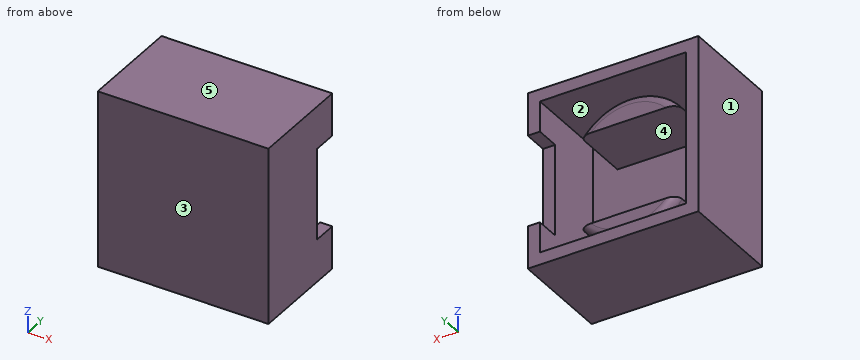
```python
from build123d import *

# Parameters (mm, degrees)
SKETCH1_W            = 30.48
SKETCH1_H            = 31.75
BOSS_EXTRUDE1_DEPTH  = 3.556
BOSS_EXTRUDE2_DEPTH  = 12.7
SKETCH4_W            = 69.596
SKETCH4_H            = 73.406
BOSS_EXTRUDE3_DEPTH  = 3.556
BOSS_EXTRUDE5_DEPTH  = 12.7
MIRROR2_COPY_1_DEPTH = 12.7
MIRROR4_COPY_1_DEPTH = 12.7
FILLET5_R            = 1.778
BOSS_EXTRUDE7_REACH  = 82.336
SKETCH9_W            = 1.524
SKETCH9_H            = 35.306
SKETCH9_H_2          = 2.794
SKETCH9_W_2          = 34.036
CUT_EXTRUDE1_DEPTH   = 81.335506123
SKETCH11_W           = 35.56
SKETCH11_H           = 36.83
SKETCH11_W_2         = 34.036
SKETCH11_H_2         = 35.306
BOSS_EXTRUDE8_DEPTH  = 16.256
BOSS_EXTRUDE9_DEPTH  = 5.08


with BuildPart() as part:
    # Sketch1 → Boss-Extrude1 (new body)
    with BuildSketch(Plane(origin=(0, 0, 0), x_dir=(1, 0, 0), z_dir=(0, 1, 0))):
        with Locations((15.24, 15.875)):
            Rectangle(SKETCH1_W, SKETCH1_H)
    extrude(amount=BOSS_EXTRUDE1_DEPTH)

    # Sketch2 → Boss-Extrude2 (add)
    with BuildSketch(Plane(origin=(0, 3.556, 0), x_dir=(1, 0, 0), z_dir=(0, 1, 0))):
        with BuildLine():
            Line((25.4, 6.35), (5.08, 6.35))
            ThreePointArc((5.08, 6.35), (15.24, 1.27), (25.4, 6.35))
        make_face()
        with BuildLine():
            ThreePointArc((25.4, 25.4), (15.24, 30.48), (5.08, 25.4))
            Line((5.08, 25.4), (25.4, 25.4))
        make_face()
    boss_extrude2 = extrude(amount=BOSS_EXTRUDE2_DEPTH)

    # Sketch4 → Boss-Extrude3 (add)
    with BuildSketch(Plane(origin=(0, 3.556, 0), x_dir=(1, 0, 0), z_dir=(0, 1, 0))):
        with Locations((33.02, -3.175)):
            Rectangle(SKETCH4_W, SKETCH4_H)
    extrude(amount=-BOSS_EXTRUDE3_DEPTH)

    # Sketch8 → Boss-Extrude5 (add)
    with BuildSketch(Plane(origin=(0, 3.556, 0), x_dir=(1, 0, 0), z_dir=(0, 1, 0))):
        Polygon((-1.778, 33.528), (-1.778, 27.178), (-1.778, 4.572), (-1.778, -1.778), (32.258, -1.778), (32.258, 33.528), align=None)
        Polygon((0, 27.178), (0, 31.75), (30.48, 31.75), (30.48, 0), (0, 0), (0, 4.572), align=None, mode=Mode.SUBTRACT)
    boss_extrude5 = extrude(amount=BOSS_EXTRUDE5_DEPTH)

    # Mirror1: Boss-Extrude5 across plane
    add(boss_extrude5.mirror(Plane(origin=(0, 0, 3.175), x_dir=(1, 0, 0), z_dir=(0, 0, -1))))

    # Mirror2: Boss-Extrude5 across plane
    add(boss_extrude5.mirror(Plane(origin=(33.02, 0, 0), x_dir=(0, 0, 1), z_dir=(1, 0, 0))))

    # Mirror2 copy 1 sketch → Mirror2 copy 1 (add)
    with BuildSketch(Plane(origin=(66.04, 3.556, 6.35), x_dir=(-1, 0, 0), z_dir=(0, 1, 0))):
        Polygon((-1.778, 33.528), (-1.778, 27.178), (-1.778, 4.572), (-1.778, -1.778), (32.258, -1.778), (32.258, 33.528), align=None)
        Polygon((0, 27.178), (0, 31.75), (30.48, 31.75), (30.48, 0), (0, 0), (0, 4.572), align=None, mode=Mode.SUBTRACT)
    extrude(amount=MIRROR2_COPY_1_DEPTH)

    # Mirror3: Boss-Extrude2 across plane
    add(boss_extrude2.mirror(Plane(origin=(0, 0, 3.175), x_dir=(1, 0, 0), z_dir=(0, 0, -1))))

    # Mirror4: Boss-Extrude2 across plane
    add(boss_extrude2.mirror(Plane(origin=(33.02, 0, 0), x_dir=(0, 0, 1), z_dir=(1, 0, 0))))

    # Mirror4 copy 1 sketch → Mirror4 copy 1 (add)
    with BuildSketch(Plane(origin=(66.04, 3.556, 6.35), x_dir=(-1, 0, 0), z_dir=(0, 1, 0))):
        with BuildLine():
            Line((25.4, 6.35), (5.08, 6.35))
            ThreePointArc((5.08, 6.35), (15.24, 1.27), (25.4, 6.35))
        make_face()
        with BuildLine():
            ThreePointArc((25.4, 25.4), (15.24, 30.48), (5.08, 25.4))
            Line((5.08, 25.4), (25.4, 25.4))
        make_face()
    extrude(amount=MIRROR4_COPY_1_DEPTH)

    # Fillet5
    fillet5_edges = [part.edges().sort_by_distance(p)[0] for p in [
        (15.24, 16.256, -1.27),
        (15.24, 16.256, 7.62),
        (15.24, 16.256, 36.83),
        (50.8, 16.256, 7.62),
        (50.8, 16.256, 36.83),
        (50.8, 16.256, -1.27),
        (50.8, 16.256, -30.48),
        (15.24, 16.256, -30.48),
    ]]
    fillet(fillet5_edges, radius=FILLET5_R)

    # Sketch9 → Boss-Extrude7 (add, up to next)
    with BuildSketch(Plane(origin=(0, 16.256, 0), x_dir=(1, 0, 0), z_dir=(0, 1, 0)), mode=Mode.PRIVATE) as boss_extrude7_sk1:
        with Locations((33.02, 15.875)):
            Rectangle(SKETCH9_W, SKETCH9_H)
    boss_extrude7_tool1 = extrude(boss_extrude7_sk1.sketch, amount=-BOSS_EXTRUDE7_REACH, mode=Mode.PRIVATE) - part.part
    # Sketch9 → Boss-Extrude7 (add, up to next)
    with BuildSketch(Plane(origin=(0, 16.256, 0), x_dir=(1, 0, 0), z_dir=(0, 1, 0)), mode=Mode.PRIVATE) as boss_extrude7_sk2:
        with Locations((33.02, -22.225)):
            Rectangle(SKETCH9_W, SKETCH9_H)
    boss_extrude7_tool2 = extrude(boss_extrude7_sk2.sketch, amount=-BOSS_EXTRUDE7_REACH, mode=Mode.PRIVATE) - part.part
    # Sketch9 → Boss-Extrude7 (add, up to next)
    with BuildSketch(Plane(origin=(0, 16.256, 0), x_dir=(1, 0, 0), z_dir=(0, 1, 0)), mode=Mode.PRIVATE) as boss_extrude7_sk3:
        with Locations((33.02, -3.175)):
            Rectangle(SKETCH9_W, SKETCH9_H_2)
    boss_extrude7_tool3 = extrude(boss_extrude7_sk3.sketch, amount=-BOSS_EXTRUDE7_REACH, mode=Mode.PRIVATE) - part.part
    # Sketch9 → Boss-Extrude7 (add, up to next)
    with BuildSketch(Plane(origin=(0, 16.256, 0), x_dir=(1, 0, 0), z_dir=(0, 1, 0)), mode=Mode.PRIVATE) as boss_extrude7_sk4:
        with Locations((50.8, -3.175)):
            Rectangle(SKETCH9_W_2, SKETCH9_H_2)
    boss_extrude7_tool4 = extrude(boss_extrude7_sk4.sketch, amount=-BOSS_EXTRUDE7_REACH, mode=Mode.PRIVATE) - part.part
    # Sketch9 → Boss-Extrude7 (add, up to next)
    with BuildSketch(Plane(origin=(0, 16.256, 0), x_dir=(1, 0, 0), z_dir=(0, 1, 0)), mode=Mode.PRIVATE) as boss_extrude7_sk5:
        with Locations((15.24, -3.175)):
            Rectangle(SKETCH9_W_2, SKETCH9_H_2)
    boss_extrude7_tool5 = extrude(boss_extrude7_sk5.sketch, amount=-BOSS_EXTRUDE7_REACH, mode=Mode.PRIVATE) - part.part
    add(boss_extrude7_tool1.solids().sort_by_distance((33.02, 16.256, -15.875))[0])
    add(boss_extrude7_tool2.solids().sort_by_distance((33.02, 16.256, 22.225))[0])
    add(boss_extrude7_tool3.solids().sort_by_distance((33.02, 16.256, 3.175))[0])
    add(boss_extrude7_tool4.solids().sort_by_distance((50.8, 16.256, 3.175))[0])
    add(boss_extrude7_tool5.solids().sort_by_distance((15.24, 16.256, 3.175))[0])

    # Sketch10 → Cut-Extrude1 (cut, through all)
    with BuildSketch(Plane(origin=(0, 16.256, 0), x_dir=(1, 0, 0), z_dir=(0, 1, 0))):
        Polygon((67.818, -4.572), (33.782, -4.572), (33.782, -39.878), (-10.061280672, -39.878), (-10.061280672, 34.690827012), (71.018790947, 34.690827012), (71.018790947, -4.572), align=None)
    extrude(amount=-CUT_EXTRUDE1_DEPTH, mode=Mode.SUBTRACT)

    # Sketch11 → Boss-Extrude8 (add)
    with BuildSketch(Plane(origin=(0, 16.256, 0), x_dir=(1, 0, 0), z_dir=(0, 1, 0))):
        with Locations((50.8, -22.225)):
            Rectangle(SKETCH11_W, SKETCH11_H)
        with Locations((50.8, -22.225)):
            Rectangle(SKETCH11_W_2, SKETCH11_H_2, mode=Mode.SUBTRACT)
    extrude(amount=-BOSS_EXTRUDE8_DEPTH)

    # Sketch12 → Boss-Extrude9 (add)
    with BuildSketch(Plane(origin=(0, 16.256, 0), x_dir=(1, 0, 0), z_dir=(0, 1, 0))):
        Polygon((66.04, -12.7), (68.58, -12.7), (68.58, -3.81), (33.02, -3.81), (33.02, -40.64), (68.58, -40.64), (68.58, -31.75), (66.04, -31.75), (66.04, -38.1), (35.56, -38.1), (35.56, -6.35), (66.04, -6.35), align=None)
    extrude(amount=BOSS_EXTRUDE9_DEPTH)


solid = part.part
```
Geometry check sheet. Reference: the model listing, model coordinates, mm. Face numbers are marked on the shaded views. A direction names the side the tool comes from. Give positions to 0.01 mm unless a question says otherwise; leave off trailing zeros. Loops run counter-clockwise (first coordinate to the right, second up) from the corner with the lowest first, then second, coordinate; pieces in that order, holes last. Notation, with made-up numbers: M -37.75,57 L 4.25,57 A29 ccw 4.25,86 Z; hole C -10.75,33.25 d7. An arc over 180 degrees is marked long. Write item = value, one per line. Start each with the question number.
1. Tool access check on the marked faces 4 and 5. Record the directions out of +Z, -Z, +X, -X, +Y, -Y that give a thin tool (end or side, any length) a straight path to the whole face; none if there is none.
2. Section check A-A, the plane y = 11.25. Enter the section's corners in (x, z), plus the area to 3 significant figures.
3. Section check D-D, the plane y = 17.5. Enter the section's corners in (x, z), plus the area to 3 significant figures.
4. Go/stop test with flat-tipped pins: P1, Ø1, axis at x = 39.5, z = 34, coming from the -Y side; P2, Ø3.5, axis at x = 53.5, z = 10.5, coming from the +Y side. Record where each tip stops, or that it passes through.
5. Section check B-B, the plane z = 15. Enter the section's corners in (x, y).
6. Section check C-C, the plane x = 37. Enter the section's corners in (y, z).
7. Thickness scan on probe 1 along X at (y, z) = (7, 18.5); probe 2 along X at (y, z) = (11.25, 11.5); probe 3 along X at (y, z) = (11, 35). Record the ranges inside material, lowest first.
8. Draft check along X on the marked faces 1, 2 and 3. Enter one of: +X half, -X half, draft (parallel to the pull), parting line (faces both ways), or undercut.
Values follow:
q1.face_4 = +Y
q1.face_5 = +Z, +X, -X, +Y, -Y
q2.outline = M 33.02,3.81 L 68.58,3.81 L 68.58,40.64 L 33.02,40.64 Z; M 40.64,12.7 A12.7 ccw 60.96,12.7 Z; M 40.64,31.75 L 60.96,31.75 A12.7 ccw Z; hole M 35.56,6.35 L 66.04,6.35 L 66.04,38.1 L 35.56,38.1 Z
q2.area = 486 mm^2
q3.outline = M 33.02,3.81 L 68.58,3.81 L 68.58,12.7 L 66.04,12.7 L 66.04,6.35 L 35.56,6.35 L 35.56,38.1 L 66.04,38.1 L 66.04,31.75 L 68.58,31.75 L 68.58,40.64 L 33.02,40.64 Z
q3.area = 294 mm^2
q4.P1 = 0
q4.P2 = 16.26
q5.outline = M 33.02,0 L 68.58,0 L 68.58,16.26 L 66.04,16.26 L 66.04,3.56 L 35.56,3.56 L 35.56,21.34 L 33.02,21.34 Z
q6.outline = M 0,3.81 L 21.34,3.81 L 21.34,6.35 L 3.56,6.35 L 3.56,38.1 L 21.34,38.1 L 21.34,40.64 L 0,40.64 Z
q7.probe_1 = 33.02 to 35.56, 66.04 to 68.58
q7.probe_2 = 33.02 to 35.56, 41.66 to 59.94, 66.04 to 68.58
q7.probe_3 = 33.02 to 35.56, 44.23 to 57.37, 66.04 to 68.58
q8.face_1 = -X half
q8.face_2 = undercut
q8.face_3 = draft
